```python
from build123d import *

# Parameters (mm, degrees)
BOSS_EXTRUDE1_DEPTH = 3
SKETCH2_W           = 3.2
SKETCH2_H           = 7.372217102
SKETCH2_H_2         = 10.2
SKETCH2_W_2         = 10.2
SKETCH2_H_3         = 3.2
CUT_EXTRUDE1_DEPTH  = 4


with BuildPart() as part:
    # Sketch1 → Boss-Extrude1 (new body)
    with BuildSketch(Plane(origin=(0, 0, 0), x_dir=(1, 0, 0), z_dir=(0, 1, 0))):
        with BuildLine():
            Line((55.172217102, -43.501443346), (55.172217102, 66.842990858))
            Line((55.172217102, 66.842990858), (-55.172217102, 66.842990858))
            Line((-55.172217102, 66.842990858), (-55.172217102, -43.501443346))
            Line((-55.172217102, -43.501443346), (-41.872217102, -43.501443346))
            ThreePointArc((-41.872217102, -43.501443346), (-38.336683196, -42.036977252), (-36.872217102, -38.501443346))
            Line((-36.872217102, -38.501443346), (-36.872217102, 48.842990858))
            ThreePointArc((-36.872217102, 48.842990858), (-36.114885762, 50.835586471), (-34.225258916, 51.822145348))
            ThreePointArc((-34.225258916, 51.822145348), (0, 53.842990858), (34.225258916, 51.822145348))
            ThreePointArc((34.225258916, 51.822145348), (36.114885762, 50.835586471), (36.872217102, 48.842990858))
            Line((36.872217102, 48.842990858), (36.872217102, -38.501443346))
            ThreePointArc((36.872217102, -38.501443346), (38.336683196, -42.036977252), (41.872217102, -43.501443346))
            Line((41.872217102, -43.501443346), (55.172217102, -43.501443346))
        make_face()
    extrude(amount=BOSS_EXTRUDE1_DEPTH)

    # Sketch2 → Cut-Extrude1 (cut, through all)
    with BuildSketch(Plane(origin=(0, 0, 0), x_dir=(1, 0, 0), z_dir=(0, 1, 0))):
        with Locations((-53.672217102, -36.915334795)):
            Rectangle(SKETCH2_W, SKETCH2_H)
        Polygon((-44.9, 63.742990858), (-44.9, 66.942990858), (-55.272217102, 66.942990858), (-55.272217102, 56.570773756), (-52.072217102, 56.570773756), (-52.072217102, 63.742990858), align=None)
        with Locations((-53.672217102, 1.670773756)):
            Rectangle(SKETCH2_W, SKETCH2_H_2)
        with Locations((-53.672217102, -18.329226244)):
            Rectangle(SKETCH2_W, SKETCH2_H_2)
        with Locations((-53.672217102, 21.670773756)):
            Rectangle(SKETCH2_W, SKETCH2_H_2)
        with Locations((-53.672217102, 41.670773756)):
            Rectangle(SKETCH2_W, SKETCH2_H_2)
        with Locations((-30, 65.342990858)):
            Rectangle(SKETCH2_W_2, SKETCH2_H_3)
        with Locations((-10, 65.342990858)):
            Rectangle(SKETCH2_W_2, SKETCH2_H_3)
        with Locations((53.672217102, 41.670773756)):
            Rectangle(SKETCH2_W, SKETCH2_H_2)
        with Locations((53.672217102, 21.670773756)):
            Rectangle(SKETCH2_W, SKETCH2_H_2)
        with Locations((53.672217102, 1.670773756)):
            Rectangle(SKETCH2_W, SKETCH2_H_2)
        with Locations((53.672217102, -18.329226244)):
            Rectangle(SKETCH2_W, SKETCH2_H_2)
        with Locations((53.672217102, -36.915334795)):
            Rectangle(SKETCH2_W, SKETCH2_H)
        with Locations((30, 65.342990858)):
            Rectangle(SKETCH2_W_2, SKETCH2_H_3)
        with Locations((10, 65.342990858)):
            Rectangle(SKETCH2_W_2, SKETCH2_H_3)
        Polygon((44.9, 66.942990858), (55.272217102, 66.942990858), (55.272217102, 56.570773756), (52.072217102, 56.570773756), (52.072217102, 63.742990858), (44.9, 63.742990858), align=None)
    extrude(amount=CUT_EXTRUDE1_DEPTH, mode=Mode.SUBTRACT)


solid = part.part
```
CAD build for the part. Positions are in the model's coordinates, mm. A direction names the side the tool comes from. Give positions to 0.01 mm unless a question says otherwise; leave off trailing zeros. Loops run counter-clockwise (first coordinate to the right, second up) from the corner with the lowest first, then second, coordinate; pieces in that order, holes last. Notation, with made-up numbers: (2, -23) -> (39, -23) arc R36 cw to (39, 14) -> close; hole circle Ø7 at (61, 34). An arc over 180 degrees is marked (long way). Use a Markdown table: item, result.
1. Slice it at A-A (z = 11). List the corners of the cut face in (x, y).
Check result:
| item | result |
|---|---|
| outline | (-55.17, 0) -> (-36.87, 0) -> (-36.87, 3) -> (-55.17, 3) -> close; (36.87, 0) -> (55.17, 0) -> (55.17, 3) -> (36.87, 3) -> close |
2. Which spindle directions (+Z, -Z, +X, -X, +Y, -Y) get a long thin tool onto all of the face, cutting with end or side? Do faces 1 (the flat face through (-54, 1, 40.601)), 2 (the flat face through (30, 1, -63.743)), 3 (the flat face through (54, 1, 3.429)), 4 (the flat face through (52.072, 1, -60)), 5 (the cylindrical face through (36.095, 1.479, -50.858)). Say none if no direction does.
Check result:
| item | result |
|---|---|
| face 1 | -X, +Y, -Y |
| face 2 | -Z, +Y, -Y |
| face 3 | +X, +Y, -Y |
| face 4 | -Z, +X, +Y, -Y |
| face 5 | +Z, +Y, -Y |
3. Mould opens along Z. For faces 6 (the flat face through (-54, 1, -56.571)), 7 (the flat face through (54, 1, 33.229)), 8 (the flat face through (-52.072, 1, -60)) say: pulls with the +Z half, pulls with the -Z half, needs draft (parallel to the pull), parting line crosses it, or undercut.
Check result:
| item | result |
|---|---|
| face 6 | pulls with the -Z half |
| face 7 | undercut |
| face 8 | needs draft |
4. Flat gauge pins, fed straight in: pin 1 (1.5 mm diameter, centred on y = 1.5, z = -21, fed in from -X); pin 2 (0.9 mm diameter, centred on y = 1.5, z = 15, fed in from +X); pin 3 (0.9 mm diameter, centred on x = -49, y = 1, fed in from -Z). Where does each tip first touch, or does it go through?
Check result:
| item | result |
|---|---|
| pin 1 | stops at x = -52.07 |
| pin 2 | stops at x = 52.07 |
| pin 3 | stops at z = -63.74 |
5. Wall check: L1, parallel to X at y = 0.8, z = 15.5; L2, parallel to X at y = 0.45, z = -13.5; L3, parallel to Z at x = 1, y = 1.4. Give the ranges that are in metal, low to high. Write a range as [from, to].
Check result:
| item | result |
|---|---|
| L1 | x = [-52.07, -36.87], [36.87, 52.07] |
| L2 | x = [-55.17, -36.87], [36.87, 55.17] |
| L3 | z = [-66.84, -53.84] |
6. Slice it at B-B (z = -44). List the corners of the cut face in (x, y), plus the area to 3 significant figures.
Check result:
| item | result |
|---|---|
| outline | (-52.07, 0) -> (-36.87, 0) -> (-36.87, 3) -> (-52.07, 3) -> close; (36.87, 0) -> (52.07, 0) -> (52.07, 3) -> (36.87, 3) -> close |
| area | 91.2 mm^2 |
7. Slice it at D-D (x = 21). List the corners of the cut face in (y, z).
Check result:
| item | result |
|---|---|
| outline | (0, -66.84) -> (3, -66.84) -> (3, -53.08) -> (0, -53.08) -> close |
8. Slice it at C-C (x = -32.5). List the corners of the cut face in (y, z), plus the area to 3 significant figures.
Check result:
| item | result |
|---|---|
| outline | (0, -63.74) -> (3, -63.74) -> (3, -52.02) -> (0, -52.02) -> close |
| area | 35.2 mm^2 |
